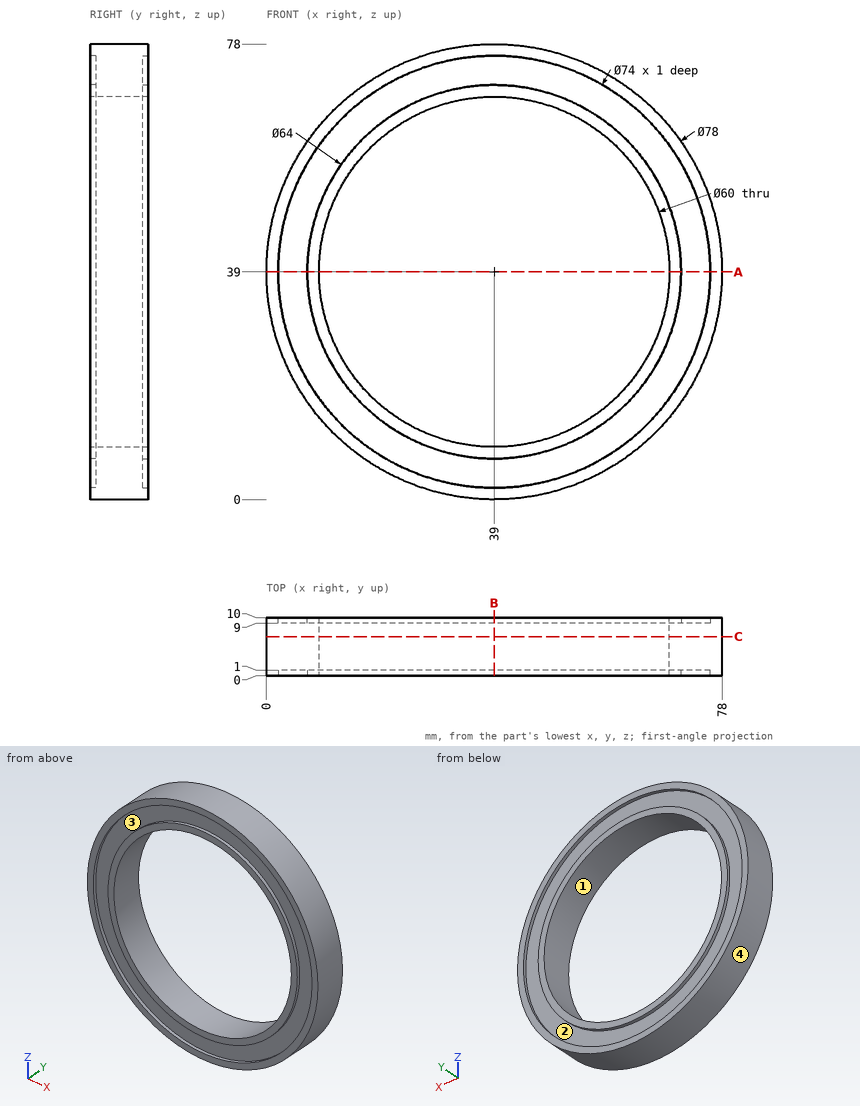
Job drawing, mm, ordinate dimensions from the low corner. One solid piece. A direction names the side the tool comes from. Coordinates: 2 decimals unless noted, no trailing zeros. Order: outer loops, then holes, each group sorted by start corner. A loop starts at its lowest first (then second) coordinate and runs counter-clockwise, first axis right, second up. Notation, with made-up numbers: (1.5, -25.75) - (5.5, -25.75) arc R22 ccw to (5.5, -15.75) - close; hole circle Ø10 at (57, 22). An arc over 180 degrees is marked (long way). Write each question's results on one line, items separated by ' | '. Start each with the question number.
Item 1: Tool access for the marked faces 1 and 2: list every direction of +Z, -Z, +X, -X, +Y, -Y with a clear straight run to the whole face (end or side of a thin tool).
Item 2: Band-saw the part on C-C on y = 6.75. Write the cut outline in (x, z), and give its area (3 significant figures).
Item 3: Flat gauge pins, fed straight in: pin 1 (1 mm diameter, centred on x = 18.5, y = 3.5, fed in from -Z); pin 2 (6 mm diameter, centred on x = 69, y = 8.5, fed in from -Z); pin 3 (6 mm diameter, centred on y = 1.5, z = 27.5, fed in from +X); pin 4 (22 mm diameter, centred on x = 23.5, z = 53.5, fed in from -Y). Where does each tip first touch, or does it go through?
Item 4: Band-saw the part on A-A on z = 39. Write the cut outline in (x, y), and give its area (3 significant figures).
Item 5: Band-saw the part on B-B on x = 39. Write the cut outline in (y, z).
Item 6: Wall check: probe 1 along Z at (x, y) = (39, 9.6); probe 2 along X at (y, z) = (0.5, 64). Give the ranges that are in metal, low to high. Write a range as [from, to].
Item 7: Mould opens along X. For the marked faces 3 and 4 say: released by +X, released by -X, zero draft, split by the parting line, or undercut.
Numbers:
1) face 1: +Y, -Y | face 2: +Y
2) outline: circle Ø78 at (39, 39); hole circle Ø60 at (39, 39) | area: 1,950 mm^2
3) pin 1: z = 5.52 | pin 2: z = 10.86 | pin 3: x = 77.06 | pin 4: y = 0
4) outline: (0, 0) - (2, 0) - (2, 1) - (7, 1) - (7, 0) - (9, 0) - (9, 10) - (7, 10) - (7, 9) - (2, 9) - (2, 10) - (0, 10) - close; (69, 0) - (71, 0) - (71, 1) - (76, 1) - (76, 0) - (78, 0) - (78, 10) - (76, 10) - (76, 9) - (71, 9) - (71, 10) - (69, 10) - close | area: 160 mm^2
5) outline: (0, 0) - (10, 0) - (10, 2) - (9, 2) - (9, 7) - (10, 7) - (10, 9) - (0, 9) - (0, 7) - (1, 7) - (1, 2) - (0, 2) - close; (0, 69) - (10, 69) - (10, 71) - (9, 71) - (9, 76) - (10, 76) - (10, 78) - (0, 78) - (0, 76) - (1, 76) - (1, 71) - (0, 71) - close
6) probe 1: [0, 2], [7, 9], [69, 71], [76, 78] | probe 2: [9.07, 11.72], [19.03, 22.42], [55.58, 58.97], [66.28, 68.93]
7) face 3: undercut | face 4: split by the parting line
